Here's the drawing with two shaded views (mm, measured from the low corner). I have some questions. A direction names the side the tool comes from. Round coordinates to 2 decimals unless told otherwise and drop trailing zeros. Order: outer loops, then holes, each group sorted by start corner. A loop starts at its lowest first (then second) coordinate and runs counter-clockwise, first axis right, second up. Notation, with made-up numbers: (36.5, 48.5) -> (44.5, 48.5) arc R25 ccw to (44.5, 74.5) -> close; hole circle Ø4 at (60.5, 41.25). An arc over 180 degrees is marked (long way). One line per question, with ' | ' between items.
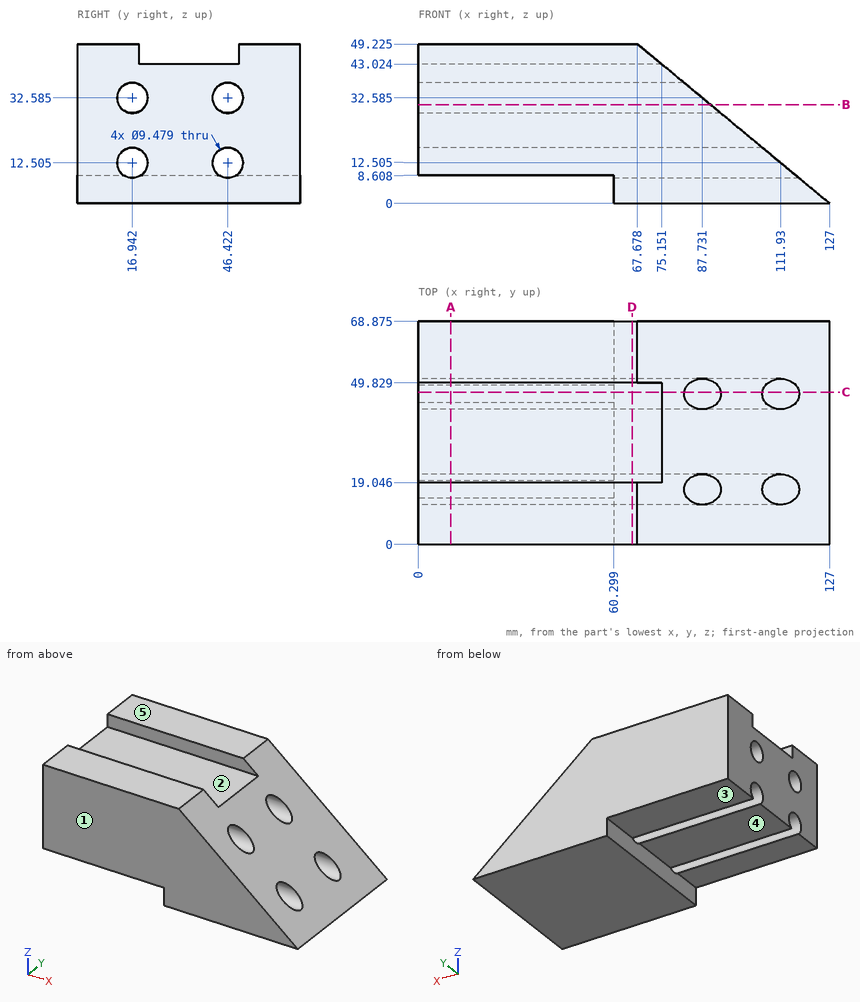
1. I want a section at B-B on z = 30.5. List the corners of the cut face in (x, y) for me (1 decimal), and give its area (3 significant figures).
From the geometry:
outline: (0, 0) -> (90.2, 0) -> (90.2, 12.7) -> (0, 12.7) -> close; (0, 21.2) -> (90.2, 21.2) -> (90.2, 42.2) -> (0, 42.2) -> close; (0, 50.7) -> (90.2, 50.7) -> (90.2, 68.9) -> (0, 68.9) -> close | area: 4,680 mm²
2. I need wall thicknesses on probe 1 along Y at (x, z) = (17.5, 13) (1 decimal); probe 2 along Z at (x, y) = (21, 50.5) (1 decimal); probe 3 along Y at (x, z) = (69, 35) (1 decimal). Which ranges of each line are inside material? Lowest first, please.
From the geometry:
probe 1: y = 0 to 12.2, 21.7 to 41.7, 51.1 to 68.9 | probe 2: z = 8.6 to 10.1, 14.9 to 30.2, 35 to 49.2 | probe 3: y = 0 to 12.9, 21 to 42.3, 50.5 to 68.9
3. I want a section at D-D on x = 66. List the corners of the cut face in (y, z) for me (1 decimal).
From the geometry:
outline: (0, 0) -> (68.9, 0) -> (68.9, 49.2) -> (49.8, 49.2) -> (49.8, 43) -> (19, 43) -> (19, 49.2) -> (0, 49.2) -> close; hole circle Ø9.5 at (16.9, 12.5); hole circle Ø9.5 at (16.9, 32.6); hole circle Ø9.5 at (46.4, 12.5); hole circle Ø9.5 at (46.4, 32.6)
4. I'm going to push flat-ended pins straight in: pin 1 (21.5 mm diameter, centred on x = 28, y = 59.5, fed in from -Z); pin 2 (3 mm diameter, centred on y = 32.5, z = 12, fed in from +X) (1 decimal); pin 3 (6 mm diameter, centred on x = 103.5, y = 40.5, fed in from +Z). Where does each tip first touch, or does it pass through?
From the geometry:
pin 1: stops at z = 8.61 | pin 2: stops at x = 114.3 | pin 3: stops at z = 21.99
5. On a 3-axis mill with a long thin cutter (end or side, diameter ignored), from which of +Z, -Z, +X, -X, +Y, -Y can I reach the whole of each face in a straight line? I mean the marked faces 4 and 5. Say none if no direction works.
From the geometry:
face 4: -Z, -X, +Y, -Y | face 5: +Z, +X, -X, +Y, -Y
6. If we mould it in two halves opening along Y, with no side actions, what happens to the marked faces 1, 2 and 3? For each: pulls with the +Y half, pulls with the -Y half, needs draft (parallel to the pull), parting line crosses it, or undercut.
From the geometry:
face 1: pulls with the -Y half | face 2: undercut | face 3: needs draft
7. I want a section at A-A on x = 10. List the corners of the cut face in (y, z) for me (1 decimal), and give its area (3 significant figures).
From the geometry:
outline: (0, 8.6) -> (14.2, 8.6) arc R4.7 cw (long way) to (19.6, 8.6) -> (43.7, 8.6) arc R4.7 cw (long way) to (49.1, 8.6) -> (68.9, 8.6) -> (68.9, 49.2) -> (49.8, 49.2) -> (49.8, 43) -> (19, 43) -> (19, 49.2) -> (0, 49.2) -> close; hole circle Ø9.5 at (16.9, 32.6); hole circle Ø9.5 at (46.4, 32.6) | area: 2,330 mm²
8. I want a section at C-C on y = 47. List the corners of the cut face in (x, z) for me, and give its area (3 significant figures).
From the geometry:
outline: (0, 17.21) -> (106.26, 17.21) -> (93.4, 27.88) -> (0, 27.88) -> close; (0, 37.29) -> (82.06, 37.29) -> (75.15, 43.02) -> (0, 43.02) -> close; (60.3, 0) -> (127, 0) -> (117.6, 7.8) -> (60.3, 7.8) -> close | area: 2,000 mm²
